For this review, take the finished solid that the model builds, in its own axes (mm). A direction names the side the tool comes from. Coordinates: 2 decimals unless noted, no trailing zeros. Write each loop counter-clockwise with the first axis right and the second up, starting at its lowest first coordinate (ties: lowest second). Pieces come first, ordered by that corner, then holes. Notation, with made-up numbers: M 51,56 L 101,56 A8 cw 101,68 Z; hole C 17.25,26.25 d10. An arc over 180 degrees is marked long. Return JSON: item names as keys, results as strings.
```python
from build123d import *

# Parameters (mm, degrees)
F_02_HEAD_DEPTH        = 7
SKETCH_3_R             = 1.5
F_03_SCREW_HOLES_DEPTH = 64.408013115
SKETCH_4_R             = 2.75
F_04_CBORE_DEPTH       = 3
SKETCH_5_R             = 3.4
F_05_M8_TAP_DEPTH      = 24


with BuildPart() as part:
    # 草图1 → 旋转1 (revolve)
    with BuildSketch(Plane.XY, mode=Mode.PRIVATE) as revolve_1_sk:
        Polygon((7, 0), (7, 9), (54, 9), (54, 8.25), (56, 8.25), (56, 9), (56.5, 9), (57, 8.5), (57, 0), align=None)
    revolve(revolve_1_sk.sketch.rotate(Axis((2, 0, 0), (1, 0, 0)), 90), axis=Axis((2, 0, 0), (1, 0, 0)))

    # 草图2 → 02_HEAD (add)
    with BuildSketch(Plane(origin=(0, 0, 0), x_dir=(0, 0, -1), z_dir=(1, 0, 0))):
        Polygon((-20, 0), (-19.96956, -0.69725), (-19.87846, -1.38919), (-19.72741, -2.07055), (-19.51754, -2.73616), (-19.25046, -3.38095), (-18.9282, -4), (-18.55322, -4.58861), (-18.12836, -5.1423), (-17.65685, -5.65685), (-17.1423, -6.12836), (-16.58861, -6.55322), (-16, -6.9282), (-15.38095, -7.25046), (-14.73616, -7.51754), (6.45637, -15.23099), (7.12198, -15.44086), (7.80335, -15.59191), (8.49529, -15.68301), (9.19253, -15.71345), (9.88978, -15.68301), (10.58172, -15.59191), (11.26309, -15.44086), (11.92869, -15.23099), (12.57348, -14.96391), (13.19253, -14.64165), (13.78114, -14.26667), (14.33483, -13.84181), (14.84939, -13.37031), (15.32089, -12.85575), (15.74575, -12.30206), (16.12074, -11.71345), (16.443, -11.0944), (16.71007, -10.44961), (16.91994, -9.784), (17.071, -9.10264), (17.16209, -8.4107), (17.19253, -7.71345), (17.16209, -7.01621), (17.071, -6.32427), (16.91994, -5.6429), (11.83165, 13.34686), (11.62178, 14.01247), (11.3547, 14.65726), (11.03244, 15.27631), (10.65746, 15.86492), (10.2326, 16.41861), (9.7611, 16.93317), (9.24654, 17.40467), (8.69285, 17.82953), (8.10424, 18.20451), (7.48519, 18.52677), (6.8404, 18.79385), (6.17479, 19.00372), (5.49343, 19.15477), (4.80149, 19.24587), (4.10424, 19.27631), (3.407, 19.24587), (2.71506, 19.15477), (2.03369, 19.00372), (1.36808, 18.79385), (0.7233, 18.52677), (0.10424, 18.20451), (-0.48437, 17.82953), (-16.58861, 6.55322), (-17.1423, 6.12836), (-17.65685, 5.65685), (-18.12836, 5.1423), (-18.55322, 4.58861), (-18.9282, 4), (-19.25046, 3.38095), (-19.51754, 2.73616), (-19.72741, 2.07055), (-19.87846, 1.38919), (-19.96956, 0.69725), align=None)
    extrude(amount=F_02_HEAD_DEPTH)

    # 草图3 → 03_SCREW_HOLES (cut, through all)
    with BuildSketch(Plane(origin=(0, 0, 0), x_dir=(0, 0, -1), z_dir=(1, 0, 0))):
        with Locations(Location((-12, 0, 0), (0, 0, 180))):
            Circle(SKETCH_3_R)
        with Locations(Location((4.10424172, 11.276311449, 0), (0, 0, 180))):
            Circle(SKETCH_3_R)
        with Locations(Location((9.192533317, -7.713451316, 0), (0, 0, 180))):
            Circle(SKETCH_3_R)
    extrude(amount=F_03_SCREW_HOLES_DEPTH, mode=Mode.SUBTRACT)

    # 草图4 → 04_CBORE (cut)
    with BuildSketch(Plane(origin=(0, 0, 0), x_dir=(0, 0, -1), z_dir=(1, 0, 0))):
        with Locations((-12, 0)):
            Circle(SKETCH_4_R)
        with Locations((4.10424172, 11.276311449)):
            Circle(SKETCH_4_R)
        with Locations((9.192533317, -7.713451316)):
            Circle(SKETCH_4_R)
    extrude(amount=F_04_CBORE_DEPTH, mode=Mode.SUBTRACT)

    # 草图5 → 05_M8_TAP (cut)
    with BuildSketch(Plane(origin=(0, 0, 0), x_dir=(0, 0, -1), z_dir=(1, 0, 0))):
        Circle(SKETCH_5_R)
    extrude(amount=F_05_M8_TAP_DEPTH, mode=Mode.SUBTRACT)


solid = part.part
```
1. Clearance check with flat-ended pins moving along their axes: pin 1 Ø3.5 at (y, z) = (11.28, -4.1) entering from -X; pin 2 Ø10 at (x, z) = (42, -10) entering from +Y; pin 3 Ø1.5 at (x, z) = (7, -1.5) entering from +Y. State where each tip first meets the part, or that it passes through.
Checks:
{"pin 1": "x = 3", "pin 2": "y = 7.48", "pin 3": "y = 19.05"}
2. We need section C-C (x = 27). State the section outline as (y, z) points, plus the area to 3 significant figures.
Checks:
{"outline": "C 0,0 d18", "area": "254 mm2"}
3. Draft analysis for pull direction Z (two halves, no side actions). For faces 5 (the face through (54, 3, 8)), 6 (the face through (3.451, 12.27, 8.424)), 7 (the face through (24, 0, 0)), state which applies: +Z half, -Z half, draft (parallel to the pull), parting line (faces both ways), or undercut.
Checks:
{"face 5": "draft", "face 6": "+Z half", "face 7": "undercut"}
4. We need section B-B (x = 21). State the section outline as (y, z) points.
Checks:
{"outline": "C 0,0 d18; hole C 0,0 d6.8"}
5. We need section A-A (z = 12). State the section outline as (x, y) points, plus the area to 3 significant figures.
Checks:
{"outline": "M 0,-8.51 L 7,-8.51 L 7,-1.5 L 3,-1.5 L 3,-2.75 L 0,-2.75 Z; M 0,2.75 L 3,2.75 L 3,1.5 L 7,1.5 L 7,9.77 L 0,9.77 Z", "area": "99.5 mm2"}
6. For faces 1 (the face through (56, 3, -8)), 2 (the face through (3, 10.1, -5.3)), 3 (the face through (30.829, -6.083, -6.633)), 4 (the face through (4.97, -8.98, -8.39)), list the 3-axis set-ups (+Z, -Z, +X, -X, +Y, -Y) from which the entire face can be reached by the end or side of a thin tool; tool diameter is ignored.
Checks:
{"face 1": "none", "face 2": "-X", "face 3": "+X", "face 4": "+X, -X"}
7. Wall thickness on L1, parallel to Y at x = 1, z = 12; L2, parallel to Y at x = 12, z = 0; L3, parallel to X at y = -13.5, z = -14: over which ranges is each line inside the solid? List them lowest first. Write a range as from..to.
Checks:
{"L1": "-8.51..-2.75, 2.75..9.77", "L2": "-9..-3.4, 3.4..9", "L3": "0..7"}
